Check sheet for the drawn part. Datum: minimum x, y, z corner. Units: mm. Coordinates: 2 decimals unless noted, no trailing zeros. Order: outer loops, then holes, each group sorted by start corner. A loop starts at its lowest first (then second) coordinate and runs counter-clockwise, first axis right, second up. Notation, with made-up numbers: (-7.5, 73.25) - (31.5, 73.25) arc R20 cw to (31.5, 93.25) - close; hole circle Ø7 at (9.25, 83.5). An arc over 180 degrees is marked (long way). Put each result on its own line as item: value.
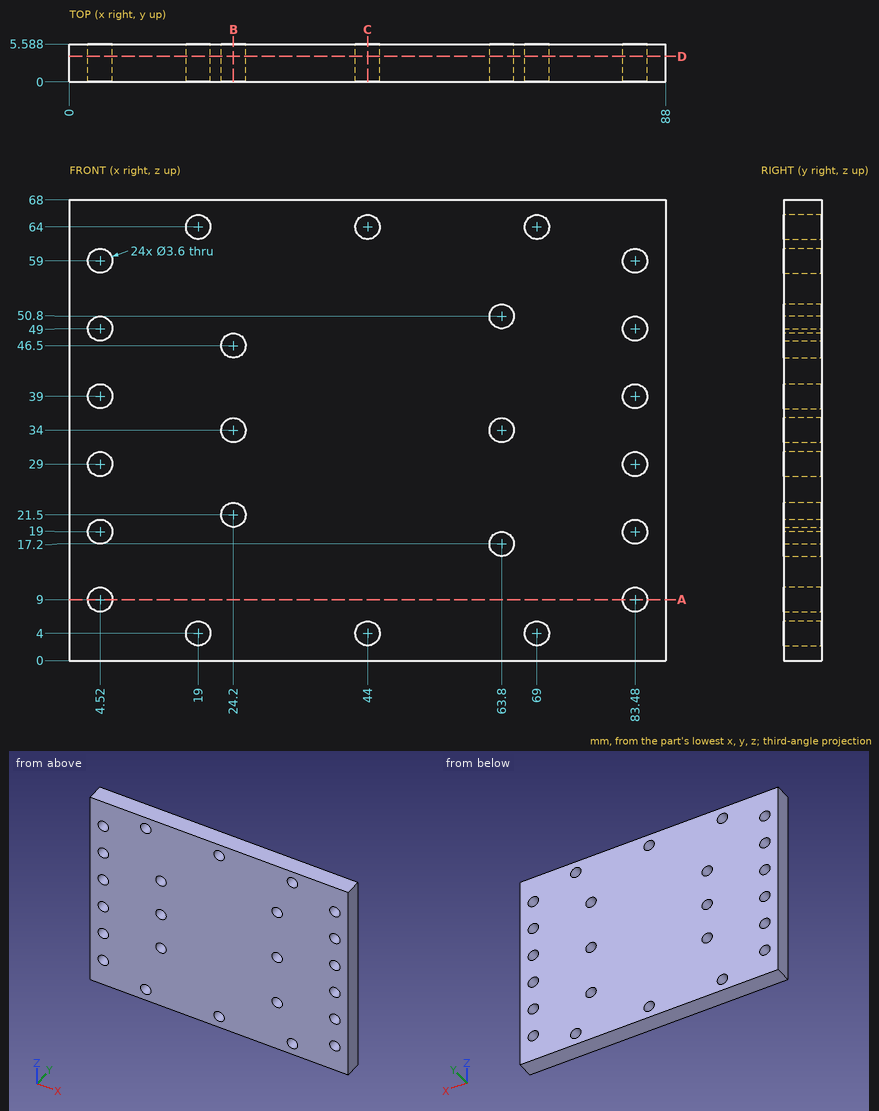
Q1. Section check B-B on x = 24.2. Record the boundary of the cut face in (y, z), then the cut area to 3 significant figures.
Answer block:
outline: (0, 0) - (5.59, 0) - (5.59, 19.7) - (0, 19.7) - close; (0, 23.3) - (5.59, 23.3) - (5.59, 32.2) - (0, 32.2) - close; (0, 35.8) - (5.59, 35.8) - (5.59, 44.7) - (0, 44.7) - close; (0, 48.3) - (5.59, 48.3) - (5.59, 68) - (0, 68) - close
area: 320 mm^2
Q2. Thickness scan on L1, parallel to X at y = 4.2, z = 64; L2, parallel to X at y = 1.25, z = 21.5; L3, parallel to X at y = 2.45, z = 39. Record the ranges inside material, lowest first. Write a range as [from, to].
Answer block:
L1: x = [0, 17.2], [20.8, 42.2], [45.8, 67.2], [70.8, 88]
L2: x = [0, 22.4], [26, 88]
L3: x = [0, 2.72], [6.32, 81.68], [85.28, 88]
Q3. Section check A-A on z = 9. Record the boundary of the cut face in (x, y).
Answer block:
outline: (0, 0) - (2.72, 0) - (2.72, 5.59) - (0, 5.59) - close; (6.32, 0) - (81.68, 0) - (81.68, 5.59) - (6.32, 5.59) - close; (85.28, 0) - (88, 0) - (88, 5.59) - (85.28, 5.59) - close
Q4. Section check C-C on x = 44. Record the boundary of the cut face in (y, z), then the cut area to 3 significant figures.
Answer block:
outline: (0, 0) - (5.59, 0) - (5.59, 2.2) - (0, 2.2) - close; (0, 5.8) - (5.59, 5.8) - (5.59, 62.2) - (0, 62.2) - close; (0, 65.8) - (5.59, 65.8) - (5.59, 68) - (0, 68) - close
area: 340 mm^2
Q5. Depth check by flat-ended pin: pin 1 Ø3 at (x, z) = (24.2, 34) entering from -Y; pin 2 Ø8 at (x, z) = (39.5, 11) entering from -Y. Enter the tip coordinate at first touch or a pass-through.
Answer block:
pin 1: passes through
pin 2: stops at y = 0
Q6. Section check D-D on y = 3.75. State how many separate pieces and enclosed holes the cut face has, then the cut area to 3 significant figures.
Answer block:
separate pieces: 1
enclosed holes: 24
area: 5,740 mm^2
